```python
from build123d import *

# Parameters (mm, degrees)
SKETCH2_R                = 15
SKETCH2_R_2              = 13.05
BOSS_EXTRUDE2_DEPTH      = 16
BOSS_EXTRUDE2_DEPTH_BACK = 8
SKETCH1_R                = 15
SKETCH1_R_2              = 9.1
BOSS_EXTRUDE3_DEPTH      = 28
SKETCH4_R                = 15
SKETCH4_R_2              = 10.9
CUT_EXTRUDE2_DEPTH       = 29
SKETCH5_W                = 6.921152332
SKETCH5_H                = 14.857061979
BOSS_EXTRUDE4_DEPTH      = 22
SKETCH3_R                = 0.75
CUT_EXTRUDE1_DEPTH       = 16
SKETCH6_R                = 15
SKETCH6_R_2              = 10.9
BOSS_EXTRUDE5_DEPTH      = 2
SKETCH7_W                = 28.232901182
SKETCH7_H                = 38.810832399
BOSS_EXTRUDE6_DEPTH      = 5.75
CUT_EXTRUDE3_DEPTH       = 8
SKETCH15_R               = 13
CUT_EXTRUDE6_DEPTH       = 5


with BuildPart() as part:
    # Sketch2 → Boss-Extrude2 (new body, two sides)
    with BuildSketch(Plane.XY.offset(3)) as boss_extrude2_sk:
        Circle(SKETCH2_R)
        Circle(SKETCH2_R_2, mode=Mode.SUBTRACT)
    extrude(amount=BOSS_EXTRUDE2_DEPTH)
    extrude(boss_extrude2_sk.sketch, amount=-BOSS_EXTRUDE2_DEPTH_BACK)

    # Sketch1 → Boss-Extrude3 (add)
    with BuildSketch(Plane.XY):
        Circle(SKETCH1_R)
        Circle(SKETCH1_R_2, mode=Mode.SUBTRACT)
    extrude(amount=BOSS_EXTRUDE3_DEPTH)

    # Sketch4 → Cut-Extrude2 (cut)
    with BuildSketch(Plane(origin=(0, 0, 0), x_dir=(-1, 0, 0), z_dir=(0, 0, -1))):
        Circle(SKETCH4_R)
        Circle(SKETCH4_R_2, mode=Mode.SUBTRACT)
    extrude(amount=-CUT_EXTRUDE2_DEPTH, mode=Mode.SUBTRACT)

    # Sketch5 → Boss-Extrude4 (add)
    with BuildSketch(Plane(origin=(10, 0, 0), x_dir=(0, 0, -1), z_dir=(1, 0, 0))):
        with Locations((0.440387125, 0.176739876)):
            Rectangle(SKETCH5_W, SKETCH5_H)
    extrude(amount=BOSS_EXTRUDE4_DEPTH)

    # Sketch3 → Cut-Extrude1 (cut, through all)
    with BuildSketch(Plane(origin=(0, 0, 0), x_dir=(1, 0, 0), z_dir=(0, 1, 0))):
        with Locations((0, -3.5)):
            Circle(SKETCH3_R)
        with Locations((0, -7.5)):
            Circle(SKETCH3_R)
        with Locations((0, -11.5)):
            Circle(SKETCH3_R)
        with Locations((0, -15.5)):
            Circle(SKETCH3_R)
        with Locations((0, -19.5)):
            Circle(SKETCH3_R)
        with Locations((0, -23.5)):
            Circle(SKETCH3_R)
    extrude(amount=-CUT_EXTRUDE1_DEPTH, mode=Mode.SUBTRACT)

    # Sketch6 → Boss-Extrude5 (add)
    with BuildSketch(Plane.XY):
        Circle(SKETCH6_R)
        Circle(SKETCH6_R_2, mode=Mode.SUBTRACT)
    extrude(amount=BOSS_EXTRUDE5_DEPTH)

    # Sketch7 → Boss-Extrude6 (add)
    with BuildSketch(Plane(origin=(32, 0, 0), x_dir=(0, 0, -1), z_dir=(1, 0, 0))):
        with Locations((0.440387125, 0.176739875)):
            Rectangle(SKETCH7_W, SKETCH7_H)
    extrude(amount=BOSS_EXTRUDE6_DEPTH)

    # Sketch9 → Cut-Extrude3 (cut)
    with BuildSketch(Plane.ZY.offset(-32)):
        with BuildLine():
            Line((-7.192763814, 16.024728338), (6.347778577, 16.024728338))
            ThreePointArc((6.347778577, 16.024728338), (9.397778577, 12.974728338), (6.347778577, 9.924728338))
            Line((6.347778577, 9.924728338), (-7.192763814, 9.924728338))
            ThreePointArc((-7.192763814, 9.924728338), (-10.242763814, 12.974728338), (-7.192763814, 16.024728338))
        make_face()
        with BuildLine():
            Line((-7.192763814, -8.96717342), (6.347778577, -8.96717342))
            ThreePointArc((6.347778577, -8.96717342), (9.397778577, -12.01717342), (6.347778577, -15.06717342))
            Line((6.347778577, -15.06717342), (-7.192763814, -15.06717342))
            ThreePointArc((-7.192763814, -15.06717342), (-10.242763814, -12.01717342), (-7.192763814, -8.96717342))
        make_face()
    extrude(amount=-CUT_EXTRUDE3_DEPTH, mode=Mode.SUBTRACT)

    # Sketch15 → Cut-Extrude6 (cut)
    with BuildSketch(Plane(origin=(0, 0, -5), x_dir=(-1, 0, 0), z_dir=(0, 0, -1))):
        Circle(SKETCH15_R)
    extrude(amount=-CUT_EXTRUDE6_DEPTH, mode=Mode.SUBTRACT)


solid = part.part
```
Source: CAD feature listing. Evaluate the final solid. Frame: model axes, mm. A direction names the side the tool comes from. Give positions to 0.01 mm unless a question says otherwise; leave off trailing zeros. Loops run counter-clockwise (first coordinate to the right, second up) from the corner with the lowest first, then second, coordinate; pieces in that order, holes last. Notation, with made-up numbers: (-31, -5) - (0, -5) arc R26 cw to (0, 30) - close; hole circle Ø10 at (74.5, 17). An arc over 180 degrees is marked (long way). Use CSV: the item, a comma, the result in double quotes. Start each with the question number.
1. Section B-B (y = 1.5). Output: boundary loops of the cut face in (x, z), then the cut area to 3 significant figures.
2. Section A-A (z = -1). Output: boundary loops of the cut face in (x, y), then the cut area to 3 significant figures.
3. Pin query (flat end, axial travel): pin 1 (0.8 mm diameter, centred on y = 6.5, z = 2.5, fed in from -X); pin 2 (1.4 mm diameter, centred on x = 0, z = 11.5, fed in from +Y); pin 3 (4.5 mm diameter, centred on x = 21.5, y = 1.5, fed in from -Z). Return the tip coordinate at first contact, or that it passes through.
4. Ray query, L1, parallel to X at y = -9.5, z = 11.5; L2, parallel to X at y = 0, z = -3.35; L3, parallel to X at y = -4, z = 5. Return the intervals inside material, ascending.
5. Reachability of faces 4 (the flat face through (35, 16.025, -1)), 5 (the cylindrical face through (-0.163, -9.972, 4.232)), 6 (the flat face through (35, 9.925, 0)), 7 (the flat face through (35, 0, -14.557)), 8 (the flat face through (35, 19.582, 0)) from +Z, -Z, +X, -X, +Y, -Y: full face, straight path, thin tool, end or side. Return the list, or none.
6. Section D-D (x = 3). Output: boundary loops of the cut face in (y, z), then the cut area to 3 significant figures.
7. Draft query along X for faces 1 (the flat face through (22, 0, -3.901)), 2 (the cylindrical face through (13, 0, -2)), 3 (the cylindrical face through (34.835, 12.908, -10.242)). Return one class per face: +X half, -X half, draft (parallel to the pull), parting line (faces both ways), or undercut.
8. Section C-C (z = 11.5). Output: boundary loops of the cut face in (x, y).
Response:
1,outline,"(-14.92, -5) - (-12.96, -5) - (-12.96, 0) - (-8.98, 0) - (-8.98, 28) - (-10.8, 28) - (-10.8, 2) - (-14.92, 2) - close; (8.98, 0) - (12.91, 0) - (12.91, -3.9) - (12.96, -3.9) - (12.96, -5) - (14.92, -5) - (14.92, -3.9) - (32, -3.9) - (32, -14.56) - (37.75, -14.56) - (37.75, 13.68) - (32, 13.68) - (32, 3.02) - (10.8, 3.02) - (10.8, 28) - (8.98, 28) - close"
1,area,"423 mm²"
2,outline,"(12.93, 7.61) arc R15 ccw (long way) to (13.13, -7.25) - (32, -7.25) - (32, -8.97) - (37.75, -8.97) - (37.75, 9.92) - (32, 9.92) - (32, 7.61) - close; (32, -19.23) - (37.75, -19.23) - (37.75, -15.07) - (32, -15.07) - close; (32, 16.02) - (37.75, 16.02) - (37.75, 19.58) - (32, 19.58) - close; hole (10.54, 7.61) - (10.6, 7.61) arc R13.05 ccw (long way) to (10.85, -7.25) - (10.79, -7.25) arc R13 ccw to start"
2,area,"588 mm²"
3,pin 1,"x = -9.03"
3,pin 2,"y = 10.9"
3,pin 3,"z = -3.9"
4,L1,"-5.34 to -0.75, 0.75 to 5.34, 32 to 37.75"
4,L2,"-15 to -13.05, 13 to 37.75"
4,L3,"-10.14 to -8.17, 8.17 to 10.14, 32 to 37.75"
5,face 4,"+X, -X"
5,face 5,"-Y"
5,face 6,"+X"
5,face 7,"-Z, +X, -X, +Y, -Y"
5,face 8,"+Z, -Z, +X, -X, +Y"
6,outline,"(-14.7, -5) - (-12.7, -5) - (-12.7, 0) - (-8.59, 0) - (-8.59, 28) - (-10.48, 28) - (-10.48, 2) - (-14.7, 2) - close; (8.59, 0) - (12.7, 0) - (12.7, -5) - (14.7, -5) - (14.7, 2) - (10.48, 2) - (10.48, 28) - (8.59, 28) - close"
6,area,"143 mm²"
7,face 1,"undercut"
7,face 2,"undercut"
7,face 3,"draft"
8,outline,"(-0.75, -10.87) - (-0.75, -9.07) arc R9.1 cw (long way) to (0.75, -9.07) - (0.75, -10.87) arc R10.9 ccw (long way) to start; (32, -19.23) - (37.75, -19.23) - (37.75, 19.58) - (32, 19.58) - close"
